Check sheet for the modelled part. Datum: model origin and axes. Units: mm. Face numbers are marked on the shaded views. A direction names the side the tool comes from. Coordinates: 2 decimals unless noted, no trailing zeros. Loops run counter-clockwise (first coordinate to the right, second up) from the corner with the lowest first, then second, coordinate; pieces in that order, holes last. Notation, with made-up numbers: M 63.5,41.5 L 97.5,41.5 A26 cw 97.5,73.5 Z; hole C -22.75,61 d10. An arc over 180 degrees is marked long. Answer in a Markdown table with one row per item. Add a question column.
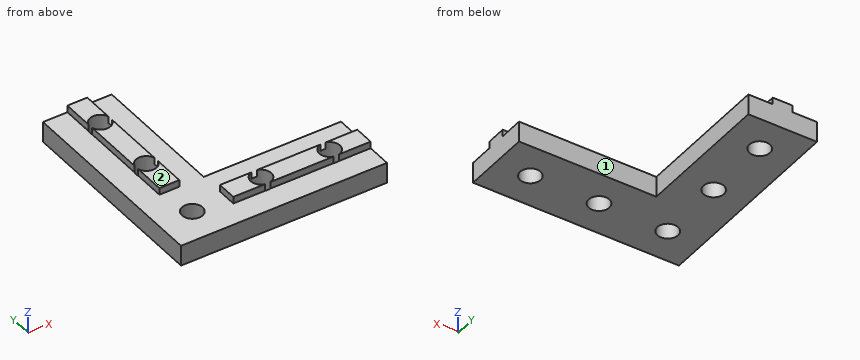
```python
from build123d import *

# Parameters (mm, degrees)
ESQUISSE1_R             = 1.5
BOSS_EXTRU_1_DEPTH      = 3
ESQUISSE2_W             = 2.9
ESQUISSE2_H             = 20
ESQUISSE2_W_2           = 20
ESQUISSE2_H_2           = 2.9
BOSS_EXTRU_2_DEPTH      = 1
ESQUISSE3_R             = 1.5
ENL_V_MAT_EXTRU_1_DEPTH = 5


with BuildPart() as part:
    # Esquisse1 → Boss.-Extru.1 (new body)
    with BuildSketch(Plane.XY):
        Polygon((0, 0), (30, 0), (30, 10), (10, 10), (10, 30), (0, 30), align=None)
        with Locations((5, 25)):
            Circle(ESQUISSE1_R, mode=Mode.SUBTRACT)
        with Locations((5, 15)):
            Circle(ESQUISSE1_R, mode=Mode.SUBTRACT)
        with Locations((5, 5)):
            Circle(ESQUISSE1_R, mode=Mode.SUBTRACT)
        with Locations((15, 5)):
            Circle(ESQUISSE1_R, mode=Mode.SUBTRACT)
        with Locations((25, 5)):
            Circle(ESQUISSE1_R, mode=Mode.SUBTRACT)
    extrude(amount=BOSS_EXTRU_1_DEPTH)

    # Esquisse2 → Boss.-Extru.2 (add)
    with BuildSketch(Plane.XY.offset(3)):
        with Locations((5, 20)):
            Rectangle(ESQUISSE2_W, ESQUISSE2_H)
        with Locations((20, 5)):
            Rectangle(ESQUISSE2_W_2, ESQUISSE2_H_2)
    extrude(amount=BOSS_EXTRU_2_DEPTH)

    # Esquisse3 → Enlèv. mat.-Extru.1 (cut, through all)
    with BuildSketch(Plane.XY.offset(4)):
        with Locations((5, 25)):
            Circle(ESQUISSE3_R)
        with Locations((5, 15)):
            Circle(ESQUISSE3_R)
        with Locations((15, 5)):
            Circle(ESQUISSE3_R)
        with Locations((25, 5)):
            Circle(ESQUISSE3_R)
    extrude(amount=-ENL_V_MAT_EXTRU_1_DEPTH, mode=Mode.SUBTRACT)


solid = part.part
```
Q1. Thickness scan on L1, parallel to Y at x = 5, z = 1.15; L2, parallel to X at y = 4.25, z = 2.7; L3, parallel to Z at x = 7, y = 5. Record the ranges inside material, lowest first.
Q2. Cross-section at B-B (z = 0.6). Record the cut outline in (x, y).
Q3. Go/stop test with flat-tipped pins: pin 1 (5 mm diameter, centred on x = 17.5, y = 10.5, fed in from -Z); pin 2 (0.5 mm diameter, centred on x = 11.5, z = 3.5, fed in from +Y); pin 3 (0.8 mm diameter, centred on x = 5, z = 3.5, fed in from -Y); pin 4 (0.5 mm diameter, centred on x = 22, z = 3.5, fed in from -Y). Record where each tip stops, or that it passes through.
Q4. Cross-section at D-D (x = 25). Record the cut outline in (y, z).
Q5. Access from +Z, -Z, +X, -X, +Y, -Y to the whole of each face (thin tool, end or side, straight path). Record for the marked faces 1 and 2.
Q6. Cross-section at A-A (x = 5). Record the cut outline in (y, z), plus the area to 3 significant figures.
Answer key:
| question | item | result |
|---|---|---|
| 1 | L1 | 0 to 3.5, 6.5 to 13.5, 16.5 to 23.5, 26.5 to 30 |
| 1 | L2 | 0 to 3.7, 6.3 to 13.7, 16.3 to 23.7, 26.3 to 30 |
| 1 | L3 | 0 to 3 |
| 2 | outline | M 0,0 L 30,0 L 30,10 L 10,10 L 10,30 L 0,30 Z; hole C 5,5 d3; hole C 5,15 d3; hole C 5,25 d3; hole C 15,5 d3; hole C 25,5 d3 |
| 3 | pin 1 | z = 0 |
| 3 | pin 2 | y = 6.45 |
| 3 | pin 3 | y = 10 |
| 3 | pin 4 | y = 3.55 |
| 4 | outline | M 0,0 L 3.5,0 L 3.5,3 L 0,3 Z; M 6.5,0 L 10,0 L 10,3 L 6.5,3 Z |
| 5 | face 1 | +Z, -Z, +X, +Y |
| 5 | face 2 | +Z, +X, -X, +Y, -Y |
| 6 | outline | M 0,0 L 3.5,0 L 3.5,3 L 0,3 Z; M 6.5,0 L 13.5,0 L 13.5,4 L 10,4 L 10,3 L 6.5,3 Z; M 16.5,0 L 23.5,0 L 23.5,4 L 16.5,4 Z; M 26.5,0 L 30,0 L 30,4 L 26.5,4 Z |
| 6 | area | 77.0 mm^2 |
